from build123d import *

# Parameters (mm, degrees)
CROQUIS3_W              = 25
CROQUIS3_H              = 35
SALIENTE_EXTRUIR2_DEPTH = 4
CROQUIS5_W              = 25
CROQUIS5_H              = 17.5
SALIENTE_EXTRUIR3_DEPTH = 2
CROQUIS7_W              = 25
CROQUIS7_H              = 10
SALIENTE_EXTRUIR5_DEPTH = 55
CROQUIS8_R              = 2.5
CORTAR_EXTRUIR1_DEPTH   = 55
SALIENTE_EXTRUIR6_DEPTH = 25
CORTAR_EXTRUIR3_DEPTH   = 4
CROQUIS11_R             = 2
CORTAR_EXTRUIR4_DEPTH   = 20
CORTAR_EXTRUIR5_DEPTH   = 45


with BuildPart() as part:
    # Croquis3 → Saliente-Extruir2 (new body)
    with BuildSketch(Plane(origin=(0, 0, 0), x_dir=(0, 0, -1), z_dir=(1, 0, 0))):
        with Locations((4.326923077, 2.8125)):
            Rectangle(CROQUIS3_W, CROQUIS3_H)
    extrude(amount=SALIENTE_EXTRUIR2_DEPTH)

    # Croquis5 → Saliente-Extruir3 (add)
    with BuildSketch(Plane(origin=(4, 0, 0), x_dir=(0, 0, -1), z_dir=(1, 0, 0))):
        with Locations((4.326923077, 11.5625)):
            Rectangle(CROQUIS5_W, CROQUIS5_H)
    extrude(amount=SALIENTE_EXTRUIR3_DEPTH)

    # Croquis7 → Saliente-Extruir5 (add)
    with BuildSketch(Plane(origin=(4, 0, 0), x_dir=(0, 0, -1), z_dir=(1, 0, 0))):
        with Locations((4.326923077, -2.1875)):
            Rectangle(CROQUIS7_W, CROQUIS7_H)
    extrude(amount=SALIENTE_EXTRUIR5_DEPTH)

    # Croquis8 → Cortar-Extruir1 (cut)
    with BuildSketch(Plane(origin=(6, 0, 0), x_dir=(0, 0, -1), z_dir=(1, 0, 0))):
        with Locations((4.326923077, 15.3125)):
            Circle(CROQUIS8_R)
        with Locations((4.326923077, 7.8125)):
            Circle(CROQUIS8_R)
    extrude(amount=-CORTAR_EXTRUIR1_DEPTH, mode=Mode.SUBTRACT)

    # Croquis10 → Saliente-Extruir6 (add, through all)
    with BuildSketch(Plane.XY.offset(8.173076923)):
        Polygon((4, -14.6875), (59, -7.1875), (4, -7.1875), align=None)
    extrude(amount=-SALIENTE_EXTRUIR6_DEPTH)

    # Croquis9 → Cortar-Extruir3 (cut)
    with BuildSketch(Plane(origin=(0, 2.8125, 0), x_dir=(1, 0, 0), z_dir=(0, 1, 0))):
        Polygon((32.505553499, 4.326923077), (28.75277675, 10.826923077), (21.24722325, 10.826923077), (17.494446501, 4.326923077), (21.24722325, -2.173076923), (28.75277675, -2.173076923), align=None)
    extrude(amount=-CORTAR_EXTRUIR3_DEPTH, mode=Mode.SUBTRACT)

    # Croquis11 → Cortar-Extruir4 (cut)
    with BuildSketch(Plane(origin=(59, 0, 0), x_dir=(0, 0, -1), z_dir=(1, 0, 0))):
        with Locations((-1.923076923, -2.1875)):
            Circle(CROQUIS11_R)
        with Locations((10.576923077, -2.1875)):
            Circle(CROQUIS11_R)
    extrude(amount=-CORTAR_EXTRUIR4_DEPTH, mode=Mode.SUBTRACT)

    # Croquis12 → Cortar-Extruir5 (cut)
    with BuildSketch(Plane(origin=(0, -1.1875, 0), x_dir=(1, 0, 0), z_dir=(0, 1, 0))):
        Polygon((30.25388745, 13.426923077), (19.74611255, 13.426923077), (14.492225101, 4.326923077), (19.74611255, -4.773076923), (30.25388745, -4.773076923), (35.507774899, 4.326923077), align=None)
    extrude(amount=-CORTAR_EXTRUIR5_DEPTH, mode=Mode.SUBTRACT)


solid = part.part
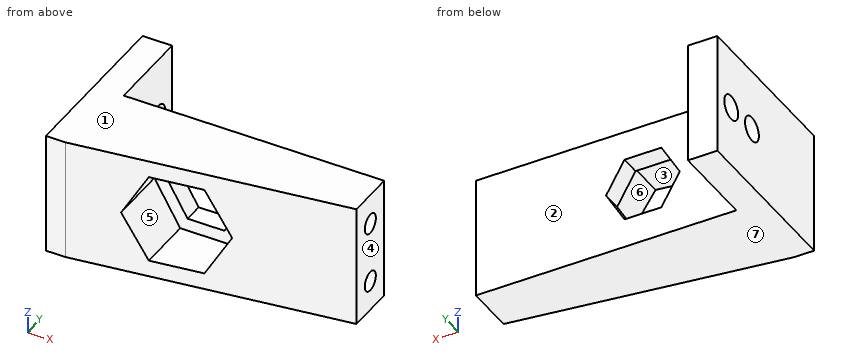
For this review, take the finished solid that the model builds, in its own axes (mm). Face numbers are marked on the shaded views. A direction names the side the tool comes from. Give positions to 0.01 mm unless a question says otherwise; leave off trailing zeros. Order: outer loops, then holes, each group sorted by start corner. A loop starts at its lowest first (then second) coordinate and runs counter-clockwise, first axis right, second up. Notation, with made-up numbers: (52, -38.5) - (92, -38.5) arc R16 cw to (92, -25.5) - close; hole circle Ø2 at (-4.75, 4). An arc over 180 degrees is marked (long way). Answer as a JSON object with one key per item and string values. Group by question number.
Item 1: Draft analysis for pull direction Z (two halves, no side actions). For the marked faces 4, 5, 6 and 7, state which applies: pulls with the +Z half, pulls with the -Z half, needs draft (parallel to the pull), parting line crosses it, or undercut.
Item 2: Take a section at D-D on y = 9. Give the boundary of the cut face in (x, z), and give its area (3 significant figures).
Item 3: Take a section at C-C on x = 24.5. Give the boundary of the cut face in (y, z).
Item 4: Clearance check with flat-ended pins moving along their axes: pin 1 Ø2 at (x, z) = (18, 2) entering from -Y; pin 2 Ø10 at (x, z) = (42, 3) entering from +Y; pin 3 Ø12 at (x, z) = (27.5, 1.5) entering from -Y. State where each tip first meets the part, or that it passes through.
Item 5: Wall thickness on line 1 along Z through (x, y) = (30, -9); line 2 along Y through (x, z) = (29, 3.25); line 3 along X through (y, z) = (12.5, 1.25): over which ranges is each line inside the solid? List them lowest first.
Item 6: Take a section at B-B on z = -9.25. Give the boundary of the cut face in (x, y), and give its area (3 significant figures).
Item 7: Take a section at A-A on y = -5. Give the boundary of the cut face in (x, z), and give its area (3 significant figures).
Item 8: Machinability: for the marked faces 1, 2 and 3, which of the approach directions +Z, -Z, +X, -X, +Y, -Y give a long, thin tool a straight path to every point of the face, cutting with its end or side? Answer none if there is none.
Reported:
{
 "1": {"face 4": "needs draft", "face 5": "undercut", "face 6": "undercut", "face 7": "pulls with the -Z half"},
 "2": {"outline": "(0, -16.83) - (6, -16.83) - (6, -6.53) - (0, -6.53) - close; (0, -2.13) - (6, -2.13) - (6, 8.17) - (0, 8.17) - close", "area": "124 mm^2"},
 "3": {"outline": "(-11.89, -16.83) - (2.81, -16.83) - (2.81, -10.83) - (-1.19, -10.83) - (-1.19, -13.43) - (-11.89, -13.43) - close; (-11.89, 4.77) - (-1.19, 4.77) - (-1.19, 2.17) - (2.81, 2.17) - (2.81, 8.17) - (-11.89, 8.17) - close"},
 "4": {"pin 1": "y = -12.91", "pin 2": "y = 2.81", "pin 3": "y = -12.17"},
 "5": {"line 1": "-16.83 to -13.43, 4.77 to 8.17", "line 2": "-1.19 to 2.81", "line 3": "0 to 6"},
 "6": {"outline": "(0, -14.69) - (4, -14.69) - (17.33, -12.87) - (17.33, -1.19) - (20.34, -1.19) - (20.34, 2.81) - (6, 2.81) - (6, 20.31) - (0, 20.31) - close; (29.66, -1.19) - (32.67, -1.19) - (32.67, -10.78) - (59, -7.19) - (59, -3.68) - (39, -3.68) - (39, -0.69) - (59, -0.69) - (59, 2.81) - (29.66, 2.81) - close", "area": "671 mm^2"},
 "7": {"outline": "(0, -16.83) - (59, -16.83) - (59, 8.17) - (0, 8.17) - close; hole (14.49, -4.33) - (19.75, -13.43) - (30.25, -13.43) - (35.51, -4.33) - (30.25, 4.77) - (19.75, 4.77) - close", "area": "1,190 mm^2"},
 "8": {"face 1": "+Z, +X, -X, +Y, -Y", "face 2": "+Z, -Z, +X, +Y", "face 3": "-Y"}
}
